from build123d import *

# Parameters (mm, degrees)
SKETCH_1_R          = 2.025
EXTRUDE_1_DEPTH     = 4
EXTRUDE_START       = -4
SKETCH_3_R          = 2.025
SKETCH_3_R_2        = 4.5
EXTRUDE_2_DEPTH     = 4
CUT_EXTRUDE_START   = -4
CUT_EXTRUDE_1_DEPTH = 4
SKETCH_5_R          = 2.025
EXTRUDE_3_DEPTH     = 4
CUT_EXTRUDE_2_DEPTH = 4
FILLET_1_R          = 5


with BuildPart() as part:
    # 草图1 → 凸台-拉伸1 (new body)
    with BuildSketch(Plane.XY):
        with BuildLine():
            Line((-136, -32.5), (136, -32.5))
            ThreePointArc((136, -32.5), (140.057826276, -29.945262427), (139.508238663, -25.181798182))
            ThreePointArc((139.508238663, -25.181798182), (131.492529199, -10.937801452), (128.498696281, 5.130179301))
            ThreePointArc((128.498696281, 5.130179301), (126.549935963, 9.641991246), (122, 11.5))
            Line((122, 11.5), (107, 11.5))
            ThreePointArc((107, 11.5), (101.988927424, 9.13994585), (100.616747965, 3.773585121))
            ThreePointArc((100.616747965, 3.773585121), (96.394657773, -12.73829458), (80.975972641, -20))
            Line((80.975972641, -20), (-80.975972641, -20))
            ThreePointArc((-80.975972641, -20), (-96.394657597, -12.738294792), (-100.616748069, 3.773584578))
            ThreePointArc((-100.616748069, 3.773584578), (-101.988927248, 9.139945637), (-107, 11.5))
            Line((-107, 11.5), (-122, 11.5))
            ThreePointArc((-122, 11.5), (-126.549935963, 9.641991246), (-128.498696281, 5.130179301))
            ThreePointArc((-128.498696281, 5.130179301), (-131.492529192, -10.937801431), (-139.508238634, -25.181798147))
            ThreePointArc((-139.508238634, -25.181798147), (-140.057826286, -29.945262407), (-136, -32.5))
        make_face()
        with Locations((-122, -28)):
            Circle(SKETCH_1_R, mode=Mode.SUBTRACT)
        with Locations((122, -5)):
            Circle(SKETCH_1_R, mode=Mode.SUBTRACT)
        with Locations((107, -5)):
            Circle(SKETCH_1_R, mode=Mode.SUBTRACT)
        with Locations((-106.75, -28)):
            Circle(SKETCH_1_R, mode=Mode.SUBTRACT)
        with Locations((-91.5, -28)):
            Circle(SKETCH_1_R, mode=Mode.SUBTRACT)
        with Locations((-76.25, -28)):
            Circle(SKETCH_1_R, mode=Mode.SUBTRACT)
        with Locations((-61, -28)):
            Circle(SKETCH_1_R, mode=Mode.SUBTRACT)
        with Locations((-45.75, -28)):
            Circle(SKETCH_1_R, mode=Mode.SUBTRACT)
        with Locations((-30.5, -28)):
            Circle(SKETCH_1_R, mode=Mode.SUBTRACT)
        with Locations((-15.25, -28)):
            Circle(SKETCH_1_R, mode=Mode.SUBTRACT)
        with Locations((0, -28)):
            Circle(SKETCH_1_R, mode=Mode.SUBTRACT)
        with Locations((15.25, -28)):
            Circle(SKETCH_1_R, mode=Mode.SUBTRACT)
        with Locations((30.5, -28)):
            Circle(SKETCH_1_R, mode=Mode.SUBTRACT)
        with Locations((45.75, -28)):
            Circle(SKETCH_1_R, mode=Mode.SUBTRACT)
        with Locations((61, -28)):
            Circle(SKETCH_1_R, mode=Mode.SUBTRACT)
        with Locations((76.25, -28)):
            Circle(SKETCH_1_R, mode=Mode.SUBTRACT)
        with Locations((91.5, -28)):
            Circle(SKETCH_1_R, mode=Mode.SUBTRACT)
        with Locations((106.75, -28)):
            Circle(SKETCH_1_R, mode=Mode.SUBTRACT)
        with Locations((-122, -5)):
            Circle(SKETCH_1_R, mode=Mode.SUBTRACT)
        with Locations((-107, -5)):
            Circle(SKETCH_1_R, mode=Mode.SUBTRACT)
        with Locations((122, -28)):
            Circle(SKETCH_1_R, mode=Mode.SUBTRACT)
        with Locations((-136, -28)):
            Circle(SKETCH_1_R, mode=Mode.SUBTRACT)
        with Locations((-122, 5)):
            Circle(SKETCH_1_R, mode=Mode.SUBTRACT)
        with Locations((136, -28)):
            Circle(SKETCH_1_R, mode=Mode.SUBTRACT)
        with Locations((-107, 5)):
            Circle(SKETCH_1_R, mode=Mode.SUBTRACT)
        with Locations((122, 5)):
            Circle(SKETCH_1_R, mode=Mode.SUBTRACT)
        with Locations((107, 5)):
            Circle(SKETCH_1_R, mode=Mode.SUBTRACT)
    extrude(amount=EXTRUDE_1_DEPTH)

    # 草图3 → 凸台-拉伸2 (add)
    # profile 1 of 3: a face of its own
    with BuildSketch(Plane.XY.offset(4).offset(EXTRUDE_START)):
        with BuildLine():
            Line((140.5, -48), (140.5, -28))
            ThreePointArc((140.5, -28), (139.181980515, -31.181980515), (136, -32.5))
            Line((136, -32.5), (-136, -32.5))
            ThreePointArc((-136, -32.5), (-139.181980515, -31.181980515), (-140.5, -28))
            Line((-140.5, -28), (-140.5, -48))
            ThreePointArc((-140.5, -48), (-136, -43.5), (-131.5, -48))
            ThreePointArc((-131.5, -48), (-132.818019485, -51.181980515), (-136, -52.5))
            Line((-136, -52.5), (136, -52.5))
            ThreePointArc((136, -52.5), (132.818019485, -44.818019485), (140.5, -48))
        make_face()
        with Locations((-122, -48)):
            Circle(SKETCH_3_R, mode=Mode.SUBTRACT)
        with Locations((-106.75, -48)):
            Circle(SKETCH_3_R, mode=Mode.SUBTRACT)
        with Locations((-91.5, -48)):
            Circle(SKETCH_3_R, mode=Mode.SUBTRACT)
        with Locations((-76.25, -48)):
            Circle(SKETCH_3_R, mode=Mode.SUBTRACT)
        with Locations((-61, -48)):
            Circle(SKETCH_3_R, mode=Mode.SUBTRACT)
        with Locations((-45.75, -48)):
            Circle(SKETCH_3_R, mode=Mode.SUBTRACT)
        with Locations((-30.5, -48)):
            Circle(SKETCH_3_R, mode=Mode.SUBTRACT)
        with Locations((-15.25, -48)):
            Circle(SKETCH_3_R, mode=Mode.SUBTRACT)
        with Locations((0, -48)):
            Circle(SKETCH_3_R, mode=Mode.SUBTRACT)
        with Locations((15.25, -48)):
            Circle(SKETCH_3_R, mode=Mode.SUBTRACT)
        with Locations((30.5, -48)):
            Circle(SKETCH_3_R, mode=Mode.SUBTRACT)
        with Locations((45.75, -48)):
            Circle(SKETCH_3_R, mode=Mode.SUBTRACT)
        with Locations((61, -48)):
            Circle(SKETCH_3_R, mode=Mode.SUBTRACT)
        with Locations((76.25, -48)):
            Circle(SKETCH_3_R, mode=Mode.SUBTRACT)
        with Locations((91.5, -48)):
            Circle(SKETCH_3_R, mode=Mode.SUBTRACT)
        with Locations((106.75, -48)):
            Circle(SKETCH_3_R, mode=Mode.SUBTRACT)
        with Locations((122, -48)):
            Circle(SKETCH_3_R, mode=Mode.SUBTRACT)
    # profile 2 of 3: a face of its own
    with BuildSketch(Plane.XY.offset(4).offset(EXTRUDE_START)):
        with Locations((-136, -48)):
            Circle(SKETCH_3_R_2)
        with Locations((-136, -48)):
            Circle(SKETCH_3_R, mode=Mode.SUBTRACT)
    # profile 3 of 3: a face of its own
    with BuildSketch(Plane.XY.offset(4).offset(EXTRUDE_START)):
        with Locations((136, -48)):
            Circle(SKETCH_3_R_2)
        with Locations((136, -48)):
            Circle(SKETCH_3_R, mode=Mode.SUBTRACT)
    extrude(amount=EXTRUDE_2_DEPTH)

    # 草图4 → 切除-拉伸1 (cut)
    with BuildSketch(Plane.XY.offset(4).offset(CUT_EXTRUDE_START)):
        with BuildLine():
            ThreePointArc((61.000988285, -20), (66.484595805, -34.784048658), (80.975972382, -41))
            ThreePointArc((80.975972382, -41), (95.118108173, -35.142135715), (100.975972641, -21))
            ThreePointArc((100.975972641, -21), (100.217086052, -15.542935341), (97.998017171, -10.5))
            ThreePointArc((97.998017171, -10.5), (90.722766985, -17.464249197), (80.975972641, -20))
            Line((80.975972641, -20), (61.000988285, -20))
        make_face()
        with BuildLine():
            ThreePointArc((97.998017171, -10.5), (76.001792969, -1.628434844), (61.000988285, -20))
            Line((61.000988285, -20), (80.975972641, -20))
            ThreePointArc((80.975972641, -20), (90.722766985, -17.464249197), (97.998017171, -10.5))
        make_face()
        with BuildLine():
            ThreePointArc((-60.975972641, -21), (-66.833837017, -35.142135624), (-80.975972641, -41))
            Line((-80.975972641, -41), (80.975972382, -41))
            ThreePointArc((80.975972382, -41), (66.484595805, -34.784048658), (61.000988285, -20))
            Line((61.000988285, -20), (-61.000988285, -20))
            ThreePointArc((-61.000988285, -20), (-60.98222753, -20.499843579), (-60.975972641, -21))
        make_face()
        with BuildLine():
            ThreePointArc((-97.998017171, -10.5), (-100.217086052, -15.542935341), (-100.975972641, -21))
            ThreePointArc((-100.975972641, -21), (-95.118108264, -35.142135624), (-80.975972641, -41))
            ThreePointArc((-80.975972641, -41), (-66.833837017, -35.142135624), (-60.975972641, -21))
            ThreePointArc((-60.975972641, -21), (-60.98222753, -20.499843579), (-61.000988285, -20))
            Line((-61.000988285, -20), (-80.975972641, -20))
            ThreePointArc((-80.975972641, -20), (-90.722766985, -17.464249197), (-97.998017171, -10.5))
        make_face()
        with BuildLine():
            ThreePointArc((-61.000988285, -20), (-76.001792969, -1.628434844), (-97.998017171, -10.5))
            ThreePointArc((-97.998017171, -10.5), (-90.722766985, -17.464249197), (-80.975972641, -20))
            Line((-80.975972641, -20), (-61.000988285, -20))
        make_face()
        with BuildLine():
            ThreePointArc((-97.998017171, -10.5), (-100.217086052, -5.457064659), (-100.975972641, 0))
            Line((-100.975972641, 0), (-100.975972641, -21))
            ThreePointArc((-100.975972641, -21), (-100.217086052, -15.542935341), (-97.998017171, -10.5))
        make_face()
        with BuildLine():
            ThreePointArc((97.998017171, -10.5), (100.217086052, -15.542935341), (100.975972641, -21))
            Line((100.975972641, -21), (100.975972641, 0))
            ThreePointArc((100.975972641, 0), (100.217086052, -5.457064659), (97.998017171, -10.5))
        make_face()
    extrude(amount=CUT_EXTRUDE_1_DEPTH, mode=Mode.SUBTRACT)

    # 草图5 → 凸台-拉伸3 (add)
    with BuildSketch(Plane.XY.offset(4).offset(EXTRUDE_START)):
        with Locations((106.75, -28)):
            Circle(SKETCH_5_R)
        with Locations((122, -28)):
            Circle(SKETCH_5_R)
        with Locations((-122, -28)):
            Circle(SKETCH_5_R)
        with Locations((-106.75, -28)):
            Circle(SKETCH_5_R)
    extrude(amount=EXTRUDE_3_DEPTH)

    # 草图6 → 切除-拉伸2 (cut)
    with BuildSketch(Plane.XY.offset(4)):
        with BuildLine():
            Line((-108.975972641, -12), (-123.395594864, -12))
            ThreePointArc((-123.395594864, -12), (-125.441584863, -17.320672039), (-128, -22.414799835))
            Line((-128, -22.414799835), (-128, -38))
            Line((-128, -38), (-108.975972641, -38))
            Line((-108.975972641, -38), (-108.975972641, -12))
        make_face()
        with BuildLine():
            Line((128, -38), (128, -22.414799835))
            ThreePointArc((128, -22.414799835), (125.441584863, -17.320672039), (123.395594864, -12))
            Line((123.395594864, -12), (108.975972641, -12))
            Line((108.975972641, -12), (108.975972641, -38))
            Line((108.975972641, -38), (128, -38))
        make_face()
    extrude(amount=-CUT_EXTRUDE_2_DEPTH, mode=Mode.SUBTRACT)

    # 圆角1
    fillet_1_edges = [part.edges().sort_by_distance(p)[0] for p in [
        (-108.975972641, -12, 2),
        (-108.975972641, -38, 2),
        (-128, -38, 2),
        (-128, -22.414799835, 2),
        (-123.395594864, -12, 2),
        (123.395594864, -12, 2),
        (128, -22.414799835, 2),
        (128, -38, 2),
        (108.975972641, -38, 2),
        (108.975972641, -12, 2),
    ]]
    fillet(fillet_1_edges, radius=FILLET_1_R)


solid = part.part
CAD build for the part. Positions are in the model's coordinates, mm. A direction names the side the tool comes from. Give positions to 0.01 mm unless a question says otherwise; leave off trailing zeros. Order: outer loops, then holes, each group sorted by start corner. A loop starts at its lowest first (then second) coordinate and runs counter-clockwise, first axis right, second up. Notation, with made-up numbers: (-2, 56) - (21, 56) arc R30 cw to (21, 87) - close; hole circle Ø6 at (81.5, 66.5). An arc over 180 degrees is marked (long way). Write each question's results on one line, items separated by ' | '.
1. Saw through at A-A on z = 2.2. Count the separate pieces of the cut face and the enclosed holes in it, and give its area (3 significant figures).
Calculated:
separate pieces: 1 | enclosed holes: 31 | area: 5,580 mm2
2. Probe L1, parallel to Y at x = -106.75, z = 1.5 (1 decimal); L2, parallel to Y at x = -118, z = 0.45; L3, parallel to Y at x = -107.5, z = 2.95. List the from-to ranges inside material, lowest first. Write a range as from..to.
Calculated:
L1: y = -52.5..-50, -46..-7, -3..3, 7..11.5 | L2: y = -52.5..-38, -12..11.5 | L3: y = -52.5..-49.88, -46.12..-6.96, -3.04..3.04, 6.96..11.5
3. Pin check, flat tips, straight feed: pin 1 (2.5 mm diameter, centred on x = 107, y = 5, fed in from -Z); pin 2 (2 mm diameter, centred on y = -23, z = 2, fed in from -X); pin 3 (2 mm diameter, centred on y = 3, z = 2, fed in from +X); pin 4 (2 mm diameter, centred on y = -3, z = 3.5, fed in from +X). Stop position of each tip, or through.
Calculated:
pin 1: passes through | pin 2: stops at x = -138.59 | pin 3: stops at x = 128.66 | pin 4: stops at x = 129.53
4. 3-axis set-ups, long thin cutter, end or side, ignore diameter. For faces 1 (the face through (110.402, -36.496, 1.972)), 2 (the face through (-126.5, 9.69, 1.97)): which of +Z, -Z, +X, -X, +Y, -Y reach the whole face in a straight line?
Calculated:
face 1: +Z, -Z | face 2: +Z, -Z, -X, +Y
5. Pull direction X, two halves, no side cores. Call faces 3 (the face through (-110.48, -13.426, 1.972)), 4 (the face through (-131.415, -10.722, 1.972)), 5 (the face through (126.6, 9.59, 1.97)), 6 (the face through (-95.27, -34.99, 1.97)): released by +X, released by -X, zero draft, split by the parting line, or undercut.
Calculated:
face 3: undercut | face 4: released by -X | face 5: released by +X | face 6: undercut
6. Saw through at B-B on x = 67. List the corners of the cut face in (y, z).
Calculated:
outline: (-52.5, 0) - (-41, 0) - (-41, 4) - (-52.5, 4) - close
